Source: CAD feature listing. Evaluate the final solid. Frame: model axes, mm. A direction names the side the tool comes from. Round coordinates to 2 decimals unless told otherwise and drop trailing zeros. Loops run counter-clockwise (first coordinate to the right, second up) from the corner with the lowest first, then second, coordinate; pieces in that order, holes last. Notation, with made-up numbers: (-17, 56.25) -> (8, 56.25) arc R23 cw to (8, 67.25) -> close; hole circle Ø2 at (22, 21.25). An arc over 180 degrees is marked (long way). Put each result on its own line as item: value. Start each with the question number.
1. Draft query along Z for faces 5 (the cylindrical face through (1.503, 11.977, -0.868)), 6 (the flat face through (5.2, -17.4, -4.2)), 7 (the flat face through (2, 0, 0)). Return one class per face: pulls with the +Z half, pulls with the -Z half, needs draft (parallel to the pull), parting line crosses it, or undercut.
2. Cut plane C-C (x = 1.1). Return the cut outline in (y, z).
3. Material intervals for L1, parallel to Z at x = 1.1, y = 12.75; L2, parallel to X at y = 16.5, z = -1.75; L3, parallel to X at y = -1.5, z = -8.25, sorted ascending.
4. Contact query for flat-ended pins moving along their axis: pin 1 (0.7 mm diameter, centred on x = 1, y = -5, fed in from -Z); pin 2 (0.8 mm diameter, centred on x = 1, z = -1.5, fed in from +Y); pin 3 (5 mm diameter, centred on y = 1, z = -9, fed in from -X); pin 4 (1.6 mm diameter, centred on x = 1, z = -1.5, fed in from -Y). Output: stop coordinate, or through.
5. Set-up query: faces 1 (the flat face through (1, 6.4, -1)), 2 (the flat face through (5, 0, -7)), 3 (the cylindrical face through (1.503, -11.977, -0.868)), 4 (the cylindrical face through (4.4, -0.24, -1.57)). Return all of +Z, -Z, +X, -X, +Y, -Y with unobstructed straight access to the full face (end or side cutting, diameter ignored); none if empty.
6. Cut plane B-B (z = -1.5). Return the cut outline in (x, y), then the cut area to 3 significant figures.
```python
from build123d import *

# Parameters (mm, degrees)
F1_DEPTH = 17.4
F2_R     = 0.75
F3_DEPTH = 11
F4_R     = 0.79999
F5_SIZE  = 0.99999


# Not quite as in the source:
# - a fillet or chamfer is up to 0.001 mm smaller than in the source, because OpenCascade refuses the exact size
# - a pattern or mirror of a feature is missing from the dataset's text; its kind, count and spacing are read off the source's solid


with BuildPart() as f1:
    # F0 (on Front) → F1 (new body, symmetric)
    with BuildSketch(Plane.XZ):
        with BuildLine():
            ThreePointArc((3, -1), (4.4142135624, -1.5857864376), (5, -3))
            Line((5, -3), (5, -12))
            Line((5, -12), (6, -12))
            Line((6, -12), (6, -3))
            ThreePointArc((6, -3), (5.1213203436, -0.8786796564), (3, 0))
            Line((3, 0), (0, 0))
            Line((0, 0), (0, -2.8))
            Line((0, -2.8), (2.2, -2.8))
            Line((2.2, -2.8), (2.2, -1))
            Line((2.2, -1), (3, -1))
        make_face()
    extrude(amount=F1_DEPTH, both=True)

    # F2 (on face) → F3 (cut)
    with BuildSketch(Plane.XZ.offset(17.4)):
        with Locations((1.1, -1.5)):
            Circle(F2_R)
    f3 = extrude(amount=-F3_DEPTH, mode=Mode.SUBTRACT)

    # F3_copies: F3 across plane
    add(f3.mirror(Plane.ZX), mode=Mode.SUBTRACT)

    # F4 (radius 0.8 in the source; OpenCascade refuses exactly that, so slightly less here)
    f4_edges = [f1.edges().sort_by_distance(p)[0] for p in [
        (2.2, 0, -1),
        (2.2, 0, -2.8),
        (0, 0, -2.8),
        (0, 0, 0),
    ]]
    fillet(f4_edges, radius=F4_R)

    # F5 (size 1 in the source; OpenCascade refuses exactly that, so slightly less here)
    f5_edges = [f1.edges().sort_by_distance(p)[0] for p in [
        (5, 0, -12),
    ]]
    chamfer(f5_edges, length=F5_SIZE)


solid = f1.part
```
Solution:
1. face 5: undercut
1. face 6: needs draft
1. face 7: pulls with the +Z half
2. outline: (-17.4, -2.8) -> (17.4, -2.8) -> (17.4, -2.25) -> (6.4, -2.25) -> (6.4, -0.75) -> (17.4, -0.75) -> (17.4, 0) -> (-17.4, 0) -> (-17.4, -0.75) -> (-6.4, -0.75) -> (-6.4, -2.25) -> (-17.4, -2.25) -> close
3. L1: z = -2.8 to -2.25, -0.75 to 0
3. L2: x = 0 to 0.39, 1.81 to 2.2, 4.56 to 5.73
3. L3: x = 5 to 6
4. pin 1: stops at z = -2.8
4. pin 2: stops at y = 6.4
4. pin 3: stops at x = 5
4. pin 4: stops at y = -17.4
5. face 1: +Y
5. face 2: -Z, -X, +Y, -Y
5. face 3: -Y
5. face 4: -Z, +Y, -Y
6. outline: (0, -17.4) -> (0.35, -17.4) -> (0.35, -6.4) -> (1.85, -6.4) -> (1.85, -17.4) -> (2.26, -17.4) -> (2.26, 17.4) -> (1.85, 17.4) -> (1.85, 6.4) -> (0.35, 6.4) -> (0.35, 17.4) -> (0, 17.4) -> close; (4.32, -17.4) -> (5.6, -17.4) -> (5.6, 17.4) -> (4.32, 17.4) -> close
6. area: 90.0 mm^2
